The listing builds one solid part. Answer for the finished solid, in the listing's coordinates (mm). Face numbers are marked on the shaded views. A direction names the side the tool comes from. Give positions to 0.01 mm unless a question says otherwise; leave off trailing zeros. Loops run counter-clockwise (first coordinate to the right, second up) from the corner with the lowest first, then second, coordinate; pieces in that order, holes last. Notation, with made-up numbers: M 63.25,-17 L 94.25,-17 A9 ccw 94.25,-10 Z; hole C 81.5,41 d8. An arc over 180 degrees is marked long. One line per item, written item: value. Start each with the question number.
Q1. A cutting plane is placed at C-C, the plane y = 13. Determine the outline of the cut face in (x, z), and give its area (3 significant figures).
Q2. The mould has two halves that part along Z. Classify the marked faces 1, 2 and 3: +Z half, -Z half, draft (parallel to the pull), parting line (faces both ways), or undercut.
Q3. Flat-ended cylindrical pins translate along their axes: pin 1 (2.5 mm diameter, centred on x = -16.5, z = 9, fed in from -Y); pin 2 (5.5 mm diameter, centred on x = -15, z = -9, fed in from -Y); pin 3 (2.5 mm diameter, centred on x = 17, z = -9, fed in from +Y). Find the tip coordinate at first contact, or state that the pin passes through.
Q4. A cutting plane is placed at A-A, the plane x = -7.5. Determine the outline of the cut face in (y, z).
Q5. A cutting plane is placed at D-D, the plane x = 39. Determine the outline of the cut face in (y, z), and give its area (3 significant figures).
Q6. A cutting plane is placed at B-B, the plane y = 9. Determine the outline of the cut face in (x, z), and give its area (3 significant figures).
Q7. For the marked faces 4, 5 and 6, determine the directions among +Z, -Z, +X, -X, +Y, -Y from which every point of the face is accessible in a straight line to the end or side of a thin tool.
Q8. Consider L1, parallel to Z at x = -7.5, y = 22.6; L2, parallel to X at y = 22, z = 9; L3, parallel to Z at x = -16.5, y = 22. Determine where each line is inside the solid, lowest interval first.
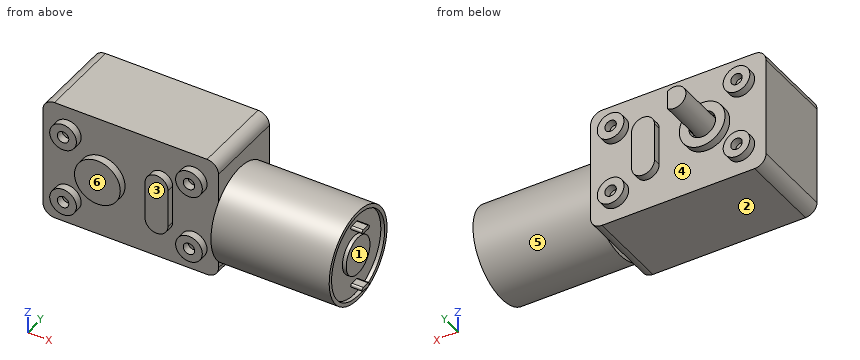
from build123d import *

# Parameters (mm, degrees)
SKETCH1_W           = 46
SKETCH1_H           = 32
BOSS_EXTRUDE1_DEPTH = 21.5
FILLET1_R           = 3
SKETCH2_R           = 3.5
SKETCH2_R_2         = 1.5
SKETCH2_R_3         = 6
BOSS_EXTRUDE2_DEPTH = 2
SKETCH3_R           = 3
BOSS_EXTRUDE3_DEPTH = 13.7
CUT_EXTRUDE1_DEPTH  = 11
SKETCH5_R           = 6
SKETCH5_R_2         = 3.5
SKETCH5_R_3         = 1.5
BOSS_EXTRUDE4_DEPTH = 2
SKETCH6_R           = 12.2
BOSS_EXTRUDE5_DEPTH = 31
SKETCH7_R           = 11.2
SKETCH7_R_2         = 5
CUT_EXTRUDE2_DEPTH  = 1
BOSS_EXTRUDE6_DEPTH = 3
CIRPATTERN1_COUNT   = 2


with BuildPart() as part:
    # Sketch1 → Boss-Extrude1 (new body)
    with BuildSketch(Plane(origin=(0, 0, 0), x_dir=(1, 0, 0), z_dir=(0, 1, 0))):
        Rectangle(SKETCH1_W, SKETCH1_H)
    extrude(amount=BOSS_EXTRUDE1_DEPTH)

    # Fillet1
    fillet1_edges = [part.edges().sort_by_distance(p)[0] for p in [
        (23, 10.75, 16),
        (-23, 10.75, 16),
        (-23, 10.75, -16),
        (23, 10.75, -16),
    ]]
    fillet(fillet1_edges, radius=FILLET1_R)

    # Sketch2 → Boss-Extrude2 (add)
    with BuildSketch(Plane(origin=(0, 21.5, 0), x_dir=(1, 0, 0), z_dir=(0, 1, 0))):
        with Locations((-16.5, 9)):
            Circle(SKETCH2_R)
        with Locations((-16.5, 9)):
            Circle(SKETCH2_R_2, mode=Mode.SUBTRACT)
        with Locations((16.5, 9)):
            Circle(SKETCH2_R)
        with Locations((16.5, 9)):
            Circle(SKETCH2_R_2, mode=Mode.SUBTRACT)
        with Locations((16.5, -9)):
            Circle(SKETCH2_R)
        with Locations((16.5, -9)):
            Circle(SKETCH2_R_2, mode=Mode.SUBTRACT)
        with Locations((-16.5, -9)):
            Circle(SKETCH2_R)
        with Locations((-16.5, -9)):
            Circle(SKETCH2_R_2, mode=Mode.SUBTRACT)
        with Locations((-7.5, 0)):
            Circle(SKETCH2_R_3)
        with Locations((-7.5, 0)):
            Circle(SKETCH2_R, mode=Mode.SUBTRACT)
        with BuildLine():
            Line((11, 5), (11, -5))
            ThreePointArc((11, -5), (8, -8), (5, -5))
            Line((5, -5), (5, 5))
            ThreePointArc((5, 5), (8, 8), (11, 5))
        make_face()
    extrude(amount=BOSS_EXTRUDE2_DEPTH)

    # Sketch3 → Boss-Extrude3 (add)
    with BuildSketch(Plane(origin=(0, 21.5, 0), x_dir=(1, 0, 0), z_dir=(0, 1, 0))):
        with Locations((-7.5, 0)):
            Circle(SKETCH3_R)
    extrude(amount=BOSS_EXTRUDE3_DEPTH)

    # Sketch4 → Cut-Extrude1 (cut)
    with BuildSketch(Plane(origin=(0, 35.2, 0), x_dir=(1, 0, 0), z_dir=(0, 1, 0))):
        Polygon((-5.7, 80.583575735), (-5.7, 2.4), (-5.7, -2.4), (-5.7, -80.583575735), (150.66715147, -80.583575735), (150.66715147, 80.583575735), align=None)
    extrude(amount=-CUT_EXTRUDE1_DEPTH, mode=Mode.SUBTRACT)

    # Sketch5 → Boss-Extrude4 (add)
    with BuildSketch(Plane.XZ):
        with Locations((-7.5, 0)):
            Circle(SKETCH5_R)
        with Locations((-16.5, -9)):
            Circle(SKETCH5_R_2)
        with Locations((-16.5, -9)):
            Circle(SKETCH5_R_3, mode=Mode.SUBTRACT)
        with Locations((-16.5, 9)):
            Circle(SKETCH5_R_2)
        with Locations((-16.5, 9)):
            Circle(SKETCH5_R_3, mode=Mode.SUBTRACT)
        with Locations((16.5, 9)):
            Circle(SKETCH5_R_2)
        with Locations((16.5, 9)):
            Circle(SKETCH5_R_3, mode=Mode.SUBTRACT)
        with Locations((16.5, -9)):
            Circle(SKETCH5_R_2)
        with Locations((16.5, -9)):
            Circle(SKETCH5_R_3, mode=Mode.SUBTRACT)
        with BuildLine():
            Line((11, -5), (11, 5))
            ThreePointArc((11, 5), (8, 8), (5, 5))
            Line((5, 5), (5, -5))
            ThreePointArc((5, -5), (8, -8), (11, -5))
        make_face()
    extrude(amount=BOSS_EXTRUDE4_DEPTH)

    # Sketch6 → Boss-Extrude5 (add)
    with BuildSketch(Plane(origin=(23, 0, 0), x_dir=(0, 0, -1), z_dir=(1, 0, 0))):
        with Locations((3, 9)):
            Circle(SKETCH6_R)
    extrude(amount=BOSS_EXTRUDE5_DEPTH)

    # Sketch7 → Cut-Extrude2 (cut)
    with BuildSketch(Plane(origin=(54, 0, 0), x_dir=(0, 0, -1), z_dir=(1, 0, 0))):
        with Locations((3, 9)):
            Circle(SKETCH7_R)
        with Locations((3, 9)):
            Circle(SKETCH7_R_2, mode=Mode.SUBTRACT)
    extrude(amount=-CUT_EXTRUDE2_DEPTH, mode=Mode.SUBTRACT)

    # Sketch8 → Boss-Extrude6 (add)
    with BuildSketch(Plane(origin=(53, 0, 0), x_dir=(0, 0, -1), z_dir=(1, 0, 0))):
        with BuildLine():
            Line((-5.5, 8), (-5.5, 10))
            ThreePointArc((-5.5, 10), (-5, 10.5), (-4.5, 10))
            Line((-4.5, 10), (-4.5, 8))
            ThreePointArc((-4.5, 8), (-5, 7.5), (-5.5, 8))
        make_face()
    boss_extrude6 = extrude(amount=BOSS_EXTRUDE6_DEPTH)

    # CirPattern1: Boss-Extrude6 ×2 about axis
    cirpattern1_axis = Axis((0, 9, -3), (1, 0, 0))
    for i in range(1, CIRPATTERN1_COUNT):
        add(boss_extrude6.rotate(cirpattern1_axis, i * 360 / CIRPATTERN1_COUNT))


solid = part.part
Answer block:
1. outline: M -23,-13 A3 ccw -20,-16 L 20,-16 A3 ccw 23,-13 L 23,-14.53 L 54,-14.53 L 54,-13.46 L 53,-13.46 L 53,-6 L 54,-6 L 54,0 L 53,0 L 53,7.46 L 54,7.46 L 54,8.53 L 23,8.53 L 23,13 A3 ccw 20,16 L -20,16 A3 ccw -23,13 Z
1. area: 2,160 mm^2
2. face 1: undercut
2. face 2: -Z half
2. face 3: draft
3. pin 1: y = 0
3. pin 2: y = -2
3. pin 3: y = 23.5
4. outline: M -2,-6 L 0,-6 L 0,-16 L 21.5,-16 L 21.5,-6 L 23.5,-6 L 23.5,-3.5 L 21.5,-3.5 L 21.5,-3 L 35.2,-3 L 35.2,3 L 21.5,3 L 21.5,3.5 L 23.5,3.5 L 23.5,6 L 21.5,6 L 21.5,16 L 0,16 L 0,6 L -2,6 Z
5. outline: C 9,-3 d24.4
5. area: 468 mm^2
6. outline: M -23,-13 A3 ccw -20,-16 L 20,-16 A3 ccw 23,-13 L 23,-15.2 L 54,-15.2 L 54,-14.2 L 53,-14.2 L 53,-11.5 L 56,-11.5 L 56,-10.5 L 53,-10.5 L 53,-8 L 54,-8 L 54,2 L 53,2 L 53,4.5 L 56,4.5 L 56,5.5 L 53,5.5 L 53,8.2 L 54,8.2 L 54,9.2 L 23,9.2 L 23,13 A3 ccw 20,16 L -20,16 A3 ccw -23,13 Z
6. area: 2,210 mm^2
7. face 4: +Y
7. face 5: +X
7. face 6: +Z, -Z, -X, -Y
8. L1: -6 to -3.5, -3 to 3, 3.5 to 6
8. L2: -20 to -18, -15 to -13, 13 to 15, 18 to 20
8. L3: -12.5 to -10.5, -7.5 to -5.5, 5.5 to 7.5, 10.5 to 12.5
